from build123d import *

# Parameters (mm, degrees)
SKETCH1_R           = 12.25
BOSS_EXTRUDE1_DEPTH = 18


with BuildPart() as part:
    # Sketch1 → Boss-Extrude1 (new body)
    with BuildSketch(Plane(origin=(0, 0, 0), x_dir=(0, 0, -1), z_dir=(1, 0, 0))):
        Polygon((0, 0), (0, 605), (180, 605), (180, 592), (1305, 400), (1305, 0), align=None)
        with Locations((1216, 365.189333333)):
            Circle(SKETCH1_R, mode=Mode.SUBTRACT)
        with Locations((1170, 373.04)):
            Circle(SKETCH1_R, mode=Mode.SUBTRACT)
    extrude(amount=BOSS_EXTRUDE1_DEPTH)


solid = part.part
Build history of the part. All positions in model axes, mm. Coordinates: 2 decimals unless noted, no trailing zeros. Order: outer loops, then holes, each group sorted by start corner. A loop starts at its lowest first (then second) coordinate and runs counter-clockwise, first axis right, second up. Notation, with made-up numbers: (34.5, 28) - (80.5, 28) arc R15 cw to (80.5, 46) - close; hole circle Ø6 at (72, -36). An arc over 180 degrees is marked (long way). Write each question's results on one line, items separated by ' | '. Start each with the question number.
Item 1: Band-saw the part on D-D on z = -726. Write the cut outline in (x, y).
Item 2: Wall check: probe 1 along Z at (x, y) = (14.75, 367); probe 2 along Y at (x, z) = (4.25, -1170); probe 3 along Y at (x, z) = (2.25, -962). Give the ranges that are in metal, low to high. Write a range as [from, to].
Item 3: Flat gauge pins, fed straight in: pin 1 (4 mm diameter, centred on x = 13.5, z = -431, fed in from -Y); pin 2 (1 mm diameter, centred on x = 7.5, z = -849.5, fed in from +Y). Where does each tip first touch, or does it go through?
Item 4: Band-saw the part on B-B on x = 9.25. Write the cut outline in (y, z), and give its area (3 significant figures).
Item 5: Band-saw the part on A-A on z = -1170. Write the cut outline in (x, y).
Item 6: Band-saw the part on C-C on z = -502.5. Write the cut outline in (x, y), and give its area (3 significant figures).
Item 7: Mould opens along Z. For faces 1 (the face through (8.87, 353.23, -1213.34)), 2 (the face through (8.874, 497.344, -734.625)), 3 (the face through (0, 240, -662)) say: released by +Z, released by -Z, zero draft, split by the parting line, or undercut.
Numbers:
1) outline: (0, 0) - (18, 0) - (18, 498.82) - (0, 498.82) - close
2) probe 1: [-1305, -1228.12], [-1203.88, -1180.66], [-1159.34, 0] | probe 2: [0, 360.79], [385.29, 423.04] | probe 3: [0, 458.54]
3) pin 1: y = 0 | pin 2: y = 477.82
4) outline: (0, -1305) - (400, -1305) - (592, -180) - (605, -180) - (605, 0) - (0, 0) - close; hole circle Ø24.5 at (365.19, -1216); hole circle Ø24.5 at (373.04, -1170) | area: 666,000 mm^2
5) outline: (0, 0) - (18, 0) - (18, 360.79) - (0, 360.79) - close; (0, 385.29) - (18, 385.29) - (18, 423.04) - (0, 423.04) - close
6) outline: (0, 0) - (18, 0) - (18, 536.96) - (0, 536.96) - close | area: 9,670 mm^2
7) face 1: undercut | face 2: released by -Z | face 3: zero draft
